```python
from build123d import *

# Parameters (mm, degrees)
F0_W     = 15.875
F0_H     = 31.75
F1_DEPTH = 4.7625
F2_R     = 2.4511
F3_DEPTH = 1.778
F4_W     = 13.462
F4_H     = 29.337
F4_R     = 3.2385
F5_DEPTH = 8.3566
F6_R     = 2.4765
F7_R     = 2.4765
F8_R     = 2.4765
F9_DEPTH = 8.3566


with BuildPart() as f1:
    # F0 (on Top) → F1 (new body, symmetric)
    with BuildSketch(Plane.XY):
        Rectangle(F0_W, F0_H)
    extrude(amount=F1_DEPTH, both=True)

    # F2 (on face) → F3 (join)
    with BuildSketch(Plane.XY.offset(4.7625)):
        with Locations((4.0132, 11.9507)):
            Circle(F2_R)
        with Locations((3.9878, 3.97514)):
            Circle(F2_R)
        with Locations((3.9878, -3.97506)):
            Circle(F2_R)
        with Locations((4.0132, -11.9507)):
            Circle(F2_R)
        with Locations((-4.0132, -11.9507)):
            Circle(F2_R)
        with Locations((-3.9878, -3.97506)):
            Circle(F2_R)
        with Locations((-3.9878, 3.97514)):
            Circle(F2_R)
        with Locations((-4.0132, 11.9507)):
            Circle(F2_R)
    extrude(amount=F3_DEPTH)

    # F4 (on face) → F5 (cut)
    with BuildSketch(Plane(origin=(0, 0, -4.7625), x_dir=(1, 0, 0), z_dir=(0, 0, -1))):
        Rectangle(F4_W, F4_H)
        with Locations((0, -7.98195)):
            Circle(F4_R, mode=Mode.SUBTRACT)
        Circle(F4_R, mode=Mode.SUBTRACT)
        with Locations((0, 7.98195)):
            Circle(F4_R, mode=Mode.SUBTRACT)
    extrude(amount=-F5_DEPTH, mode=Mode.SUBTRACT)

    # F6 (on face) + F7 (on face) + F8 (on face) → F9 (cut)
    with BuildSketch(Plane(origin=(0, 0, -4.7625), x_dir=(1, 0, 0), z_dir=(0, 0, -1))):
        Circle(F6_R)
    with BuildSketch(Plane(origin=(0, 0, -4.7625), x_dir=(1, 0, 0), z_dir=(0, 0, -1))):
        with Locations((0, 7.98195)):
            Circle(F7_R)
    with BuildSketch(Plane(origin=(0, 0, -4.7625), x_dir=(1, 0, 0), z_dir=(0, 0, -1))):
        with Locations((0, -7.98195)):
            Circle(F8_R)
    extrude(amount=-F9_DEPTH, mode=Mode.SUBTRACT)


solid = f1.part
```
Geometry check sheet. Reference: the model listing, model coordinates, mm. A direction names the side the tool comes from. Coordinates: 2 decimals unless noted, no trailing zeros. Order: outer loops, then holes, each group sorted by start corner. A loop starts at its lowest first (then second) coordinate and runs counter-clockwise, first axis right, second up. Notation, with made-up numbers: M -3.75,-25 L 47.25,-25 A35 cw 47.25,14 Z; hole C -4.75,85.5 d7. An arc over 180 degrees is marked long. One line per question, with ' | ' between items. Start each with the question number.
Item 1: Cross-section at B-B on z = 5.5. Enter the section's corners in (x, y), then the cut area to 3 significant figures.
Item 2: Draft check along X on faces 1 (the cylindrical face through (-4.545, -14.344, 5.639)), 2 (the flat face through (-4, 4, 6.54)). Enter one of: pulls with the +X half, pulls with the -X half, needs draft (parallel to the pull), parting line crosses it, or undercut.
Item 3: Gauge pin test, flat ends, axial feed: pin 1 (4 mm diameter, centred on x = 0, y = 0, fed in from +Z); pin 2 (1.5 mm diameter, centred on x = -1, y = 9, fed in from -Z). Record the tip position at first contact, or that the pin passes through.
Item 4: Cross-section at D-D on y = 0. Enter the section's corners in (x, z), then the cut area to 3 significant figures.
Item 5: Cross-section at A-A on z = 1. Enter the section's corners in (x, y) (1 decimal).
Item 6: Material ranges on L1, parallel to X at y = 0, z = 1.5; L2, parallel to Y at x = -4.75, z = -1.5 (1 decimal); L3, parallel to X at y = -1, z = 3.5, recorded low to high. Write a range as [from, to].
Item 7: Set-up check for faces 3 (the flat face through (4, 12, 6.54)), 4 (the flat face through (0, 8, 3.594)), 5 (the cylindrical face through (3.482, -14.344, 5.639)): record each of +Z, -Z, +X, -X, +Y, -Y from which the full face is reachable in a straight line by a thin tool's end or side.
Findings:
1) outline: C -4.01,-11.95 d4.9; C -4.01,11.95 d4.9; C -3.99,-3.98 d4.9; C -3.99,3.98 d4.9; C 3.99,-3.98 d4.9; C 3.99,3.98 d4.9; C 4.01,-11.95 d4.9; C 4.01,11.95 d4.9 | area: 151 mm²
2) face 1: undercut | face 2: needs draft
3) pin 1: stops at z = 4.76 | pin 2: stops at z = 3.59
4) outline: M -7.94,-4.76 L -6.73,-4.76 L -6.73,3.59 L -3.24,3.59 L -3.24,-4.76 L -2.48,-4.76 L -2.48,3.59 L 2.48,3.59 L 2.48,-4.76 L 3.24,-4.76 L 3.24,3.59 L 6.73,3.59 L 6.73,-4.76 L 7.94,-4.76 L 7.94,4.76 L -7.94,4.76 Z | area: 51.4 mm²
5) outline: M -7.9,-15.9 L 7.9,-15.9 L 7.9,15.9 L -7.9,15.9 Z; C 0,-8 d6.5; C 0,0 d6.5; C 0,8 d6.5; hole M -6.7,-14.7 L 6.7,-14.7 L 6.7,14.7 L -6.7,14.7 Z; hole C 0,-8 d5; hole C 0,0 d5; hole C 0,8 d5
6) L1: x = [-7.94, -6.73], [-3.24, -2.48], [2.48, 3.24], [6.73, 7.94] | L2: y = [-15.9, -14.7], [14.7, 15.9] | L3: x = [-7.94, -6.73], [-3.08, -2.27], [2.27, 3.08], [6.73, 7.94]
7) face 3: +Z, +X, -X, +Y, -Y | face 4: -Z | face 5: +Z
